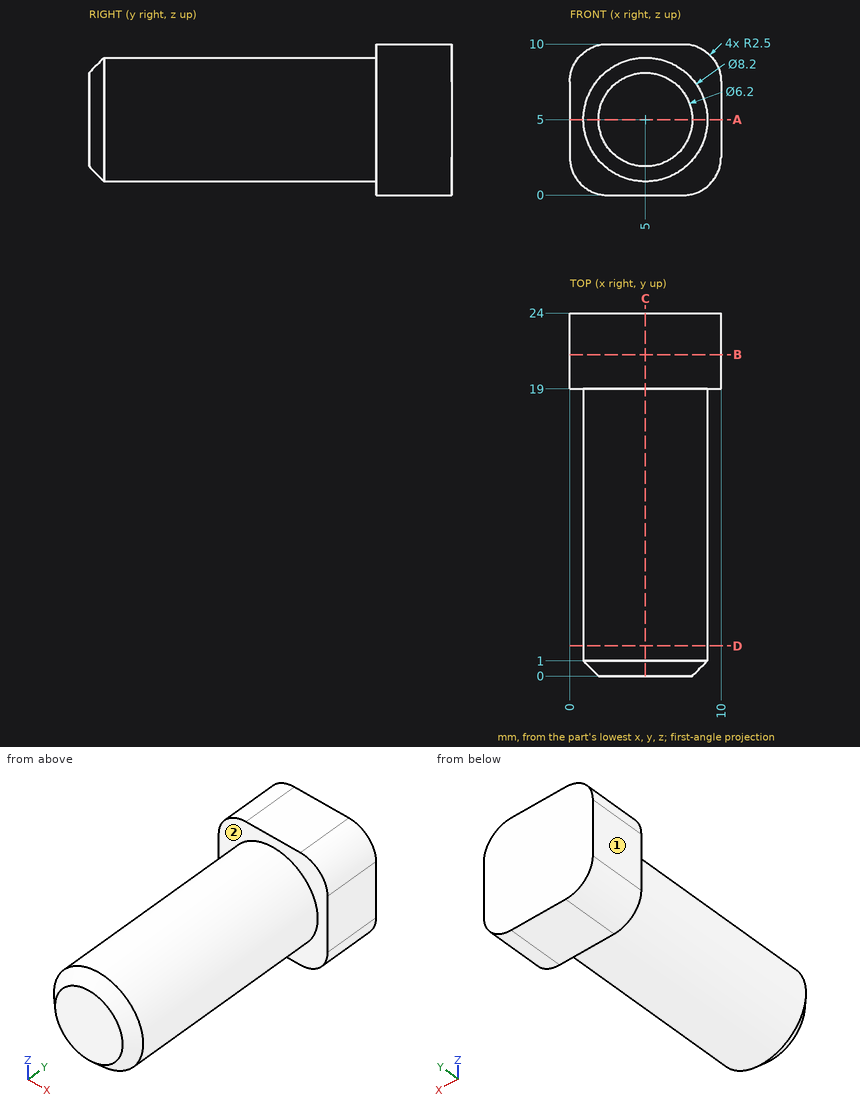
Part print with two shaded views. Sizes in mm from the minimum x, y, z corner. A direction names the side the tool comes from. Round coordinates to 2 decimals unless told otherwise and drop trailing zeros. Loops run counter-clockwise (first coordinate to the right, second up) from the corner with the lowest first, then second, coordinate; pieces in that order, holes last.
Item 1: Saw through at B-B (y = 21.25). List the corners of the cut face in (x, z), then the cut area to 3 significant figures.
Item 2: Which spindle directions (+Z, -Z, +X, -X, +Y, -Y) get a long thin tool onto all of the face, cutting with end or side? Do the marked faces 1 and 2. Say none if no direction does.
Item 3: Pin check, flat tips, straight feed: P1, Ø5, axis at x = 6, z = 2.5, coming from the -Y side; P2, Ø1.5, axis at x = 4.5, y = 14, coming from the -Z side; P3, Ø6, axis at y = 7.5, z = 3, coming from the +X side; P4, Ø1.5, axis at x = 2, y = 15.5, coming from the -Z side. Stop position of each tip, or through.
Item 4: Saw through at C-C (x = 5). List the corners of the cut face in (y, z), then the cut area to 3 significant figures.
Item 5: Drill centre lines: line 1 along Y through (x, z) = (1.25, 9.5); line 2 along Y through (x, z) = (5.5, 1.5); line 3 along X through (y, z) = (17.5, 5). Where is each one in solid material? Low to high.
Item 6: Saw through at A-A (z = 5). List the corners of the cut face in (x, y), then the cut area to 3 significant figures.
Item 7: Saw through at D-D (y = 2). List the corners of the cut face in (x, z), then the cut area to 3 significant figures.
Worked answers:
1. outline: (0, 2.5) arc R2.5 ccw to (2.5, 0) - (7.5, 0) arc R2.5 ccw to (10, 2.5) - (10, 7.5) arc R2.5 ccw to (7.5, 10) - (2.5, 10) arc R2.5 ccw to (0, 7.5) - close
1. area: 94.6 mm2
2. face 1: +Z, -Z, -X, +Y, -Y
2. face 2: -Y
3. P1: stops at y = 0
3. P2: stops at z = 0.9
3. P3: stops at x = 9.1
3. P4: stops at z = 1.57
4. outline: (0, 1.9) - (1, 0.9) - (19, 0.9) - (19, 0) - (24, 0) - (24, 10) - (19, 10) - (19, 9.1) - (1, 9.1) - (0, 8.1) - close
4. area: 205 mm2
5. line 1: y = 19 to 24
5. line 2: y = 0.44 to 24
5. line 3: x = 0.9 to 9.1
6. outline: (0, 19) - (0.9, 19) - (0.9, 1) - (1.9, 0) - (8.1, 0) - (9.1, 1) - (9.1, 19) - (10, 19) - (10, 24) - (0, 24) - close
6. area: 205 mm2
7. outline: circle Ø8.2 at (5, 5)
7. area: 52.8 mm2
